Check sheet for the drawn part. Datum: minimum x, y, z corner. Units: mm. A direction names the side the tool comes from. Round coordinates to 2 decimals unless told otherwise and drop trailing zeros. Write each loop counter-clockwise with the first axis right and the second up, starting at its lowest first coordinate (ties: lowest second). Pieces come first, ordered by that corner, then holes. Notation, with made-up numbers: M 65.25,32.25 L 87.25,32.25 A21 cw 87.25,40.25 Z; hole C 3.5,86 d3. An arc over 180 degrees is marked long. Use a Markdown table: item, result.
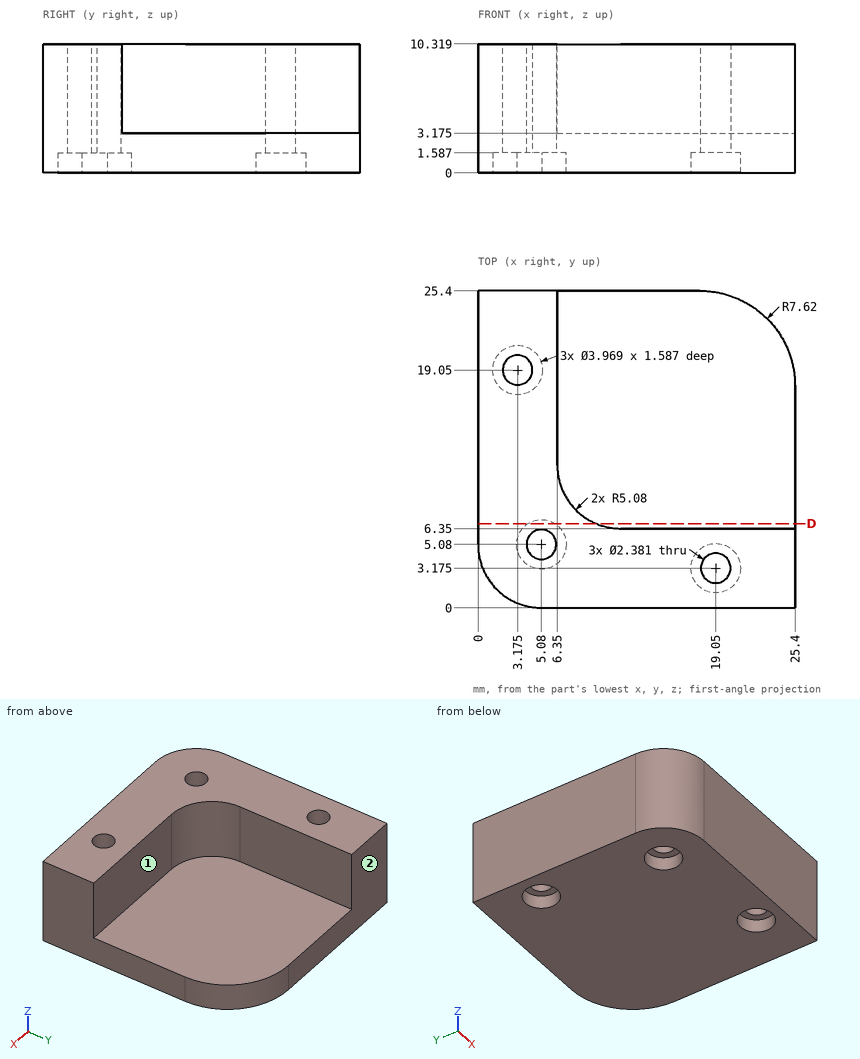
Item 1: Go/stop test with flat-tipped pins: pin 1 (6.5 mm diameter, centred on x = 19.05, y = 3.175, fed in from +Z); pin 2 (2 mm diameter, centred on x = 14, z = 8, fed in from +Y); pin 3 (3.5 mm diameter, centred on x = 5.08, y = 5.08, fed in from -Z); pin 4 (5 mm diameter, centred on x = 10.5, z = 6, fed in from +Y). Record where each tip stops, or that it passes through.
Outcome:
| item | result |
|---|---|
| pin 1 | stops at z = 10.32 |
| pin 2 | stops at y = 6.35 |
| pin 3 | stops at z = 1.59 |
| pin 4 | stops at y = 7.68 |
Item 2: Cross-section at D-D, the plane y = 6.75. Record the cut outline in (x, z) (1 decimal).
Outcome:
| item | result |
|---|---|
| outline | M 0,0 L 4,0 L 4,1.6 L 6.2,1.6 L 6.2,0 L 25.4,0 L 25.4,3.2 L 9.5,3.2 L 9.5,10.3 L 0,10.3 Z |
Item 3: Material ranges on line 1 along Y through (x, z) = (5.08, 8.25); line 2 along Y through (x, z) = (16, 7.5); line 3 along Z through (x, y) = (3.75, 4), recorded low to high. Write a range as from..to.
Outcome:
| item | result |
|---|---|
| line 1 | y = 0..3.89, 6.27..25.4 |
| line 2 | y = 0..6.35 |
| line 3 | z = 1.59..10.32 |
Item 4: Access from +Z, -Z, +X, -X, +Y, -Y to the whole of each face (thin tool, end or side, straight path). Record for the marked faces 1 and 2.
Outcome:
| item | result |
|---|---|
| face 1 | +Z, +X, +Y |
| face 2 | +Z, -Z, +X, -X, +Y |
